Answer from the drawing. Dimensions are ordinates in mm from the lowest x, y and z of the part. Give positions to 0.01 mm unless a question says otherwise; leave off trailing zeros. Order: outer loops, then holes, each group sorted by start corner. A loop starts at its lowest first (then second) coordinate and runs counter-clockwise, first axis right, second up. Notation, with made-up numbers: M -17.5,-18 L 14.5,-18 A24 ccw 14.5,-7 Z; hole C 3.5,37.5 d8. An arc over 180 degrees is marked long. One line per item, written item: value.
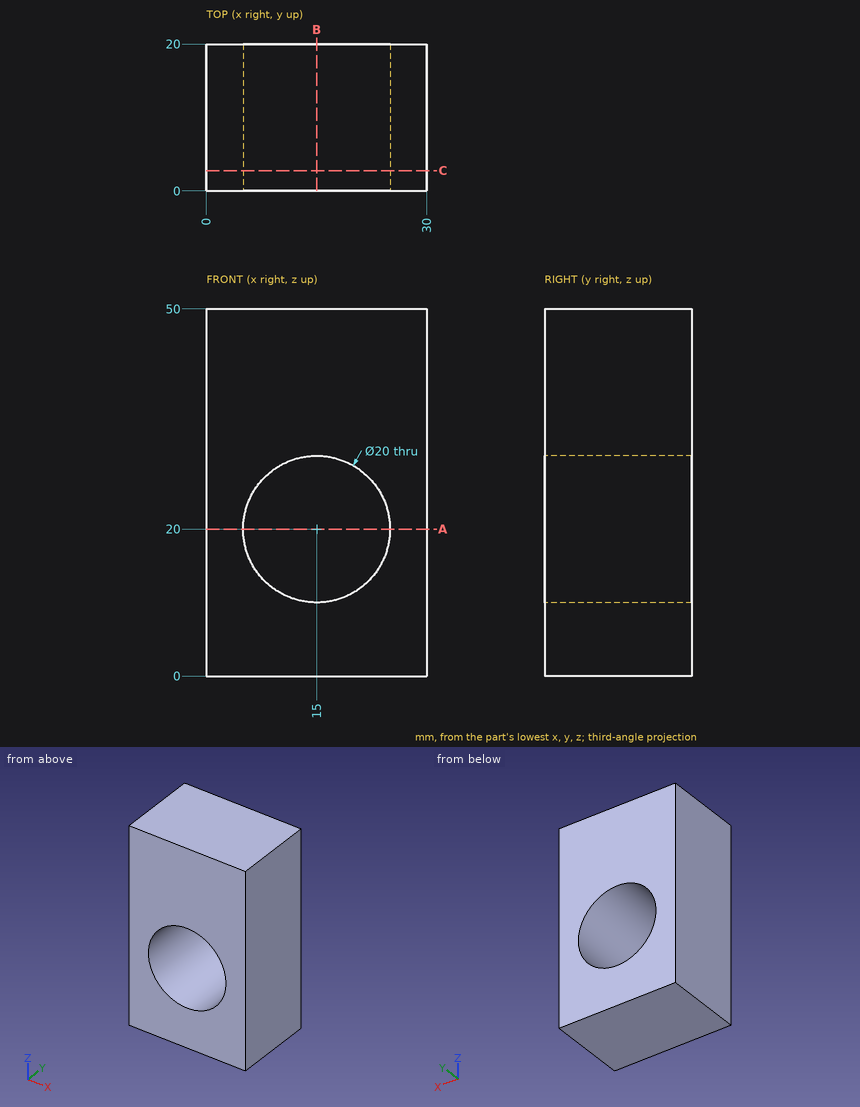
(1) Section A-A, the plane z = 20 is taken. Give the vertices of the cut face in (x, y), then the cut area to 3 significant figures.
Findings:
outline: M 0,0 L 5,0 L 5,20 L 0,20 Z; M 25,0 L 30,0 L 30,20 L 25,20 Z
area: 200 mm^2
(2) Find the intervals of material crossed by probe 1 along X at (y, z) = (15.75, 20); probe 2 along Z at (x, y) = (15, 7.75); probe 3 along Z at (x, y) = (17, 14), in increasing order. Write a range as from..to.
Findings:
probe 1: x = 0..5, 25..30
probe 2: z = 0..10, 30..50
probe 3: z = 0..10.2, 29.8..50
(3) Section B-B, the plane x = 15 is taken. Give the vertices of the cut face in (y, z), then the cut area to 3 significant figures.
Findings:
outline: M 0,0 L 20,0 L 20,10 L 0,10 Z; M 0,30 L 20,30 L 20,50 L 0,50 Z
area: 600 mm^2
(4) Given P1, Ø18, axis at x = 15, z = 20, coming from the -Y side, flat-ended and moving along its own axis, determine where the tip first touches the part or whether it passes through.
Findings:
P1: passes through
(5) Section C-C, the plane y = 2.75 is taken. Give the vertices of the cut face in (x, z).
Findings:
outline: M 0,0 L 30,0 L 30,50 L 0,50 Z; hole C 15,20 d20
